Part model, mm, in its own coordinate system. A direction names the side the tool comes from. Coordinates: 2 decimals unless noted, no trailing zeros. Loops run counter-clockwise (first coordinate to the right, second up) from the corner with the lowest first, then second, coordinate; pieces in that order, holes last.
```python
from build123d import *

# Parameters (mm, degrees)
BOSS_EXTRUDE2_DEPTH = 2.1082
BOSS_EXTRUDE3_DEPTH = 0.9
SKETCH13_W          = 8.400608993
SKETCH13_H          = 1.5
BOSS_EXTRUDE4_DEPTH = 12.7
SKETCH16_W          = 7.09322036
SKETCH16_H          = 1.5
BOSS_EXTRUDE5_DEPTH = 11.8
BOSS_EXTRUDE6_DEPTH = 2.1082
BOSS_EXTRUDE7_REACH = 45.656
BOSS_EXTRUDE8_DEPTH = 2.1082
FILLET1_R           = 6.35
SKETCH20_R          = 2.794
CUT_EXTRUDE1_DEPTH  = 46.30015706
SKETCH21_R          = 4.572
CUT_EXTRUDE2_DEPTH  = 46.30015706
BOSS_EXTRUDE9_REACH = 47.612


with BuildPart() as part:
    # Sketch6 → Boss-Extrude2 (new body)
    with BuildSketch(Plane(origin=(0, 0, 0), x_dir=(1, 0, 0), z_dir=(0, 1, 0))):
        with BuildLine():
            Line((3.1496, 3.175), (3.1496, 8.27377964))
            Line((3.1496, 8.27377964), (-5.741348421, 8.27377964))
            Line((-5.741348421, 8.27377964), (-8.59506403, 5.42006403))
            ThreePointArc((-8.59506403, 5.42006403), (-9.283317516, 4.390019898), (-9.525, 3.175))
            Line((-9.525, 3.175), (-9.525, -1.92377964))
            Line((-9.525, -1.92377964), (-6.989909723, -1.92377964))
            Line((-6.989909723, -1.92377964), (3.1496, -1.92377964))
            Line((3.1496, -1.92377964), (3.1496, 3.175))
        make_face()
    extrude(amount=BOSS_EXTRUDE2_DEPTH)

    # Sketch7 → Boss-Extrude3 (add)
    with BuildSketch(Plane.XZ):
        with BuildLine():
            Line((-2.050608993, 1.92377964), (-2.050608993, 0.42377964))
            ThreePointArc((-2.050608993, 0.42377964), (-0.881374643, -4.411978027), (-4.017957094, -8.27377964))
            Line((-4.017957094, -8.27377964), (6.35, -8.27377964))
            ThreePointArc((6.35, -8.27377964), (11.44877964, -3.175), (6.35, 1.92377964))
            Line((6.35, 1.92377964), (-2.050608993, 1.92377964))
        make_face()
    extrude(amount=BOSS_EXTRUDE3_DEPTH)

    # Sketch11 → Revolve4 (revolve)
    with BuildSketch(Plane.XY.offset(-3.175), mode=Mode.PRIVATE) as revolve4_sk:
        with BuildLine():
            Line((6.35, -0.9), (6.35, -2.083581452))
            ThreePointArc((6.35, -2.083581452), (7.929346537, -1.776499661), (9.278562256, -0.9))
            Line((9.278562256, -0.9), (6.35, -0.9))
        make_face()
    revolve(revolve4_sk.sketch.rotate(Axis((6.35, -0.9, -3.175), (0, -1, 0)), 180), axis=Axis((6.35, -0.9, -3.175), (0, -1, 0)))

    # Sketch12 → Cut-Revolve1 (revolve, cut)
    with BuildSketch(Plane.XY.offset(-3.175), mode=Mode.PRIVATE) as cut_revolve1_sk:
        with BuildLine():
            Line((8.89, 0), (6.35, 0))
            Line((6.35, 0), (6.35, -1.184421452))
            ThreePointArc((6.35, -1.184421452), (7.751289957, -0.873762947), (8.89, 0))
        make_face()
    revolve(cut_revolve1_sk.sketch.rotate(Axis((6.35, 0, -3.175), (0, -1, 0)), 180), axis=Axis((6.35, 0, -3.175), (0, -1, 0)), mode=Mode.SUBTRACT)

    # Sketch13 → Boss-Extrude4 (add)
    with BuildSketch(Plane.XZ):
        with Locations((2.149695504, 1.17377964)):
            Rectangle(SKETCH13_W, SKETCH13_H)
    extrude(amount=BOSS_EXTRUDE4_DEPTH)

    # Sketch16 → Boss-Extrude5 (add)
    with BuildSketch(Plane.XZ.offset(0.9)):
        with Locations((2.80338982, -7.52377964)):
            Rectangle(SKETCH16_W, SKETCH16_H)
    extrude(amount=BOSS_EXTRUDE5_DEPTH)

    # Mirror1: part across plane


with BuildPart() as part_1:
    add(part.part)
    add(part.part.mirror(Plane(origin=(6.35, -12.7, 1.92377964), x_dir=(0, 0, 1), z_dir=(0, 1, 0))))

    # Sketch17 → Boss-Extrude6 (add)
    with BuildSketch(Plane.XZ.offset(27.5082)):
        with BuildLine():
            Line((-5.741348421, -8.27377964), (-34.925, 1.92377964))
            Line((-34.925, 1.92377964), (-9.525, 1.92377964))
            Line((-9.525, 1.92377964), (-9.525, -3.175))
            ThreePointArc((-9.525, -3.175), (-9.283317516, -4.390019898), (-8.59506403, -5.42006403))
            Line((-8.59506403, -5.42006403), (-5.741348421, -8.27377964))
        make_face()
    extrude(amount=-BOSS_EXTRUDE6_DEPTH)

    # Boss-Extrude7: up to this face of the body (flat: up to its plane)
    boss_extrude7_end = Plane(part_1.part.faces().sort_by_distance((-20.33317421, -26.4541, -3.175))[0])
    # Sketch18 → Boss-Extrude7 (add, up to the picked face)
    with BuildSketch(Plane.ZY.offset(2.050608993), mode=Mode.PRIVATE) as boss_extrude7_sk1:
        Polygon((1.92377964, 0), (0.42377964, 0), (0.42377964, -0.9), (0.42377964, -24.5), (0.42377964, -25.4), (1.92377964, -25.4), align=None)
    boss_extrude7_tool1 = split(extrude(boss_extrude7_sk1.sketch, amount=BOSS_EXTRUDE7_REACH, mode=Mode.PRIVATE), bisect_by=boss_extrude7_end, keep=Keep.BOTH, mode=Mode.PRIVATE)
    add(boss_extrude7_tool1.solids().sort_by(Axis((-2.050609, -12.7, 1.17378), (-1, 0, 0)))[0])

    # Sketch19 → Boss-Extrude8 (add)
    with BuildSketch(Plane(origin=(0, 2.1082, 0), x_dir=(1, 0, 0), z_dir=(0, 1, 0))):
        with BuildLine():
            Line((-5.741348421, 8.27377964), (-30.632259338, -0.42377964))
            Line((-30.632259338, -0.42377964), (-9.525, -0.42377964))
            Line((-9.525, -0.42377964), (-9.525, 3.175))
            ThreePointArc((-9.525, 3.175), (-9.283317516, 4.390019898), (-8.59506403, 5.42006403))
            Line((-8.59506403, 5.42006403), (-5.741348421, 8.27377964))
        make_face()
        Polygon((-9.525, -0.42377964), (-30.632259338, -0.42377964), (-34.925, -1.92377964), (-9.525, -1.92377964), align=None)
    extrude(amount=-BOSS_EXTRUDE8_DEPTH)

    # Fillet1
    fillet1_edges = [part_1.edges().sort_by_distance(p)[0] for p in [
        (-5.741348421, 1.0541, -8.27377964),
        (-5.741348421, -26.4541, -8.27377964),
    ]]
    fillet(fillet1_edges, radius=FILLET1_R)

    # Sketch20 → Cut-Extrude1 (cut, through all)
    with BuildSketch(Plane(origin=(0, 0, 0.42377964), x_dir=(-1, 0, 0), z_dir=(0, 0, -1))):
        with Locations((18.415, -22.86)):
            Circle(SKETCH20_R)
        with Locations((18.415, -2.54)):
            Circle(SKETCH20_R)
    extrude(amount=-CUT_EXTRUDE1_DEPTH, mode=Mode.SUBTRACT)

    # Sketch21 → Cut-Extrude2 (cut, through all)
    with BuildSketch(Plane(origin=(0, 0, 0.42377964), x_dir=(-1, 0, 0), z_dir=(0, 0, -1))):
        with Locations((18.415, -22.86)):
            Circle(SKETCH21_R)
        with Locations((18.415, -2.54)):
            Circle(SKETCH21_R)
    extrude(amount=CUT_EXTRUDE2_DEPTH, mode=Mode.SUBTRACT)

    # Boss-Extrude9: up to this plane
    boss_extrude9_end = Plane(origin=(-5.741348421, 5.514005479, -8.27377964), z_dir=(-0.3298685861491406, 0, -0.9440268618381402))
    # Sketch22 → Boss-Extrude9 (add, up to the surface)
    with BuildSketch(Plane.XY.offset(1.92377964), mode=Mode.PRIVATE) as boss_extrude9_sk1:
        with BuildLine():
            Line((-14.088715594, -27.5082), (-22.741284406, -27.5082))
            ThreePointArc((-22.741284406, -27.5082), (-18.415, -29.21), (-14.088715594, -27.5082))
        make_face()
    boss_extrude9_tool1 = split(extrude(boss_extrude9_sk1.sketch, amount=-BOSS_EXTRUDE9_REACH, mode=Mode.PRIVATE), bisect_by=boss_extrude9_end, keep=Keep.BOTH, mode=Mode.PRIVATE)
    add(boss_extrude9_tool1.solids().sort_by_distance((-18.415, -28.197399, 1.92378))[0])
    # Sketch22 → Boss-Extrude9 (add, up to the surface)
    with BuildSketch(Plane.XY.offset(1.92377964), mode=Mode.PRIVATE) as boss_extrude9_sk2:
        with BuildLine():
            Line((-22.741284406, 2.1082), (-14.088715594, 2.1082))
            ThreePointArc((-14.088715594, 2.1082), (-18.415, 3.81), (-22.741284406, 2.1082))
        make_face()
    boss_extrude9_tool2 = split(extrude(boss_extrude9_sk2.sketch, amount=-BOSS_EXTRUDE9_REACH, mode=Mode.PRIVATE), bisect_by=boss_extrude9_end, keep=Keep.BOTH, mode=Mode.PRIVATE)
    add(boss_extrude9_tool2.solids().sort_by_distance((-18.415, 2.797399, 1.92378))[0])


solid = part_1.part
```
Q1. Tool access for faces 4 (the flat face through (-8, -25.4, -3)), 5 (the flat face through (-25, 0, 0)), 6 (the flat face through (3, -13, -6.774)), 7 (the flat face through (3.6, -0.9, -5.4)): list every direction of +Z, -Z, +X, -X, +Y, -Y with a clear straight run to the whole face (end or side of a thin tool).
Q2. Drop flat-ended pins along their axis: P1, Ø1.1, axis at y = -27, z = -4.5, coming from the +X side; P2, Ø3, axis at x = -25.5, z = -1.5, coming from the +Y side; P3, Ø6.5, axis at x = -18.415, y = -22.86, coming from the -Z side; P4, Ø1, axis at x = -17, z = -6.5, coming from the +Y side. Give the stop position or say it passes through.
Q3. Probe line 1 (Z direction, x = 0, y = -1.5); line 2 (Y direction, x = 2, z = -1); line 3 (Y direction, x = 7, z = 0.5). List the from-to ranges inside material, lowest first.
Q4. Mould opens along Z. For faces 1 (the flat face through (-27, -27.508, 0)), 2 (the cylindrical face through (-0.866, -24.956, -4.341)), 3 (the cylindrical face through (11.448, -24.956, -3.287)) say: released by +Z, released by -Z, zero draft, split by the parting line, or undercut.
Q5. Saw through at B-B (y = -9). List the corners of the cut face in (x, z) (3 decimals), plus the area to 3 significant figures.
Q6. Saw through at D-D (x = -29.5). List the corners of the cut face in (y, z), plus the area to 3 significant figures.
Q7. Saw through at A-A (x = 1.5). List the corners of the cut face in (y, z), plus the area to 3 significant figures.
Checked values:
1. face 4: -X
1. face 5: -Z, -X
1. face 6: +X, -X
1. face 7: none
2. P1: stops at x = 3.15
2. P2: stops at y = 2.11
2. P3: stops at z = 0.42
2. P4: passes through
3. line 1: z = -8.27 to -6.77, 0.42 to 1.92
3. line 2: y = -27.51 to -24.5, -0.9 to 2.11
3. line 3: y = -25.4 to -24.5, -0.9 to 0
4. face 1: zero draft
4. face 2: undercut
4. face 3: split by the parting line
5. outline: (-34.925, 1.924) - (-30.632, 0.424) - (6.35, 0.424) - (6.35, 1.924) - close; (-0.743, -8.274) - (6.35, -8.274) - (6.35, -6.774) - (-0.743, -6.774) - close
5. area: 69.3 mm2
6. outline: (-27.51, 0.03) - (-25.4, 0.03) - (-25.4, 0.42) - (0, 0.42) - (0, 0.03) - (2.11, 0.03) - (2.11, 1.92) - (-27.51, 1.92) - close
6. area: 46.1 mm2
7. outline: (-27.51, -8.27) - (2.11, -8.27) - (2.11, 1.92) - (-27.51, 1.92) - close; hole (-24.5, -6.77) - (-0.9, -6.77) - (-0.9, 0.42) - (-24.5, 0.42) - close
7. area: 132 mm2
